from build123d import *

# Parameters (mm, degrees)
SKETCH_2_R      = 31.5
SKETCH_2_R_2    = 30.249929249
EXTRUDE_1_DEPTH = 2


with BuildPart() as part:
    # 草图1 → 旋转1 (revolve)
    with BuildSketch(Plane.XY, mode=Mode.PRIVATE) as revolve_1_sk:
        Polygon((-31.978791145, 45), (-31.5, 0), (-30.249929249, 0), (-30.75, 47), (-32.45, 47), (-32.45, 45), align=None)
    revolve(revolve_1_sk.sketch.rotate(Axis((0, -2.4, 0), (0, 1, 0)), 270), axis=Axis((0, -2.4, 0), (0, 1, 0)))

    # 草图2 → 凸台-拉伸1 (add)
    with BuildSketch(Plane.XZ):
        with Locations(Location((0, 0, 0), (0, 0, 270))):
            Circle(SKETCH_2_R)
        with Locations(Location((0, 0, 0), (0, 0, 270))):
            Circle(SKETCH_2_R_2, mode=Mode.SUBTRACT)
    extrude(amount=EXTRUDE_1_DEPTH)


solid = part.part
Work out the finished part from the listing and answer in its coordinate system (mm). A direction names the side the tool comes from. Give positions to 0.01 mm unless a question says otherwise; leave off trailing zeros. Loops run counter-clockwise (first coordinate to the right, second up) from the corner with the lowest first, then second, coordinate; pieces in that order, holes last. Notation, with made-up numbers: (49.5, -18.75) -> (96.5, -18.75) arc R19 cw to (96.5, 2.25) -> close; hole circle Ø10 at (73, 39). An arc over 180 degrees is marked (long way). Use a Markdown table: item, result. Add a question column.
1) Each of these flat-tipped pins is pushed along its axis until it touches: P1, Ø8, axis at x = -7.5, y = 36, coming from the -Z side; P2, Ø2, axis at x = 16, y = 39, coming from the -Z side; P3, Ø1.5, axis at y = 27, z = -20, coming from the -X side. Where does it stop, or does it pass through?
2) The part is cut by section A-A, the plane y = 19.5. Determine the outline of the cut face in (x, z), plus the area to 3 significant figures.
3) For a pull along Z with two mould halves and no side action, classify faces 1 (the flat face through (21.5, 45, -23.9)), 2 (the conical face through (18.561, 23.829, 24.207)), 3 (the conical face through (30.98, 22.18, 6.88)) as +Z half, -Z half, draft (parallel to the pull), parting line (faces both ways), or undercut.
4) Consider line 1 along Z through (x, y) = (0, -1); line 2 along X through (y, z) = (20, 3.5). Determine where each line is inside the solid, lowest interval first.
5) The part is cut by section B-B, the plane y = 34. Determine the outline of the cut face in (x, z).
6) Which of the six approach directions +Z, -Z, +X, -X, +Y, -Y give full straight-line access (tool end or side, diameter ignored) to faces 4 (the flat face through (12, -2, 28)), 5 (the cylindrical face through (31.232, -0.986, 4.101))?
Reported:
| question | item | result |
|---|---|---|
| 1 | P1 | stops at z = -31.69 |
| 1 | P2 | stops at z = -28.17 |
| 1 | P3 | stops at x = -25.3 |
| 2 | outline | circle Ø63.41 at (0, 0); hole circle Ø60.91 at (0, 0) |
| 2 | area | 244 mm^2 |
| 3 | face 1 | draft |
| 3 | face 2 | undercut |
| 3 | face 3 | parting line |
| 4 | line 1 | z = -31.5 to -30.25, 30.25 to 31.5 |
| 4 | line 2 | x = -31.52 to -30.26, 30.26 to 31.52 |
| 5 | outline | circle Ø63.72 at (0, 0); hole circle Ø61.22 at (0, 0) |
| 6 | face 4 | +Z, -Z, +X, -X, -Y |
| 6 | face 5 | -Y |
